from build123d import *

# Parameters (mm, degrees)
F1_DEPTH = 1600
F2_R     = 4.5
F3_DEPTH = 40.001


with BuildPart() as f1:
    # F0 (on Top) → F1 (new body)
    with BuildSketch(Plane.XY):
        with BuildLine():
            Line((-15.5, -20), (15.5, -20))
            ThreePointArc((15.5, -20), (18.681981, -18.681981), (20, -15.5))
            Line((20, -15.5), (20, 15.5))
            ThreePointArc((20, 15.5), (18.681981, 18.681981), (15.5, 20))
            Line((15.5, 20), (-15.5, 20))
            ThreePointArc((-15.5, 20), (-18.681981, 18.681981), (-20, 15.5))
            Line((-20, 15.5), (-20, -15.5))
            ThreePointArc((-20, -15.5), (-18.681981, -18.681981), (-15.5, -20))
        make_face()
        with BuildLine():
            ThreePointArc((15.5, 17), (16.56066, 16.56066), (17, 15.5))
            Line((17, 15.5), (17, -15.5))
            ThreePointArc((17, -15.5), (16.56066, -16.56066), (15.5, -17))
            Line((15.5, -17), (-15.5, -17))
            ThreePointArc((-15.5, -17), (-16.56066, -16.56066), (-17, -15.5))
            Line((-17, -15.5), (-17, 15.5))
            ThreePointArc((-17, 15.5), (-16.56066, 16.56066), (-15.5, 17))
            Line((-15.5, 17), (15.5, 17))
        make_face(mode=Mode.SUBTRACT)
    extrude(amount=F1_DEPTH)

    # F2 (on face) → F3 (cut, through all)
    with BuildSketch(Plane.YZ.offset(20)):
        with Locations((0, 1540)):
            Circle(F2_R)
        with Locations((0, 60)):
            Circle(F2_R)
    extrude(amount=-F3_DEPTH, mode=Mode.SUBTRACT)


solid = f1.part
Check sheet for the modelled part. Datum: model origin and axes. Units: mm. A direction names the side the tool comes from. Give positions to 0.01 mm unless a question says otherwise; leave off trailing zeros. Loops run counter-clockwise (first coordinate to the right, second up) from the corner with the lowest first, then second, coordinate; pieces in that order, holes last. Notation, with made-up numbers: M 38,57 L 81,57 A21 cw 81,91 Z; hole C 84,-34 d7. An arc over 180 degrees is marked long. Answer as a JSON object with one key per item and string values. Group by question number.
Q1. Cross-section at A-A on x = 8.5. Record the cut outline in (y, z), then the cut area to 3 significant figures.
Q2. Material ranges on line 1 along Z through (x, y) = (17.9, 0); line 2 along X through (y, z) = (-5, 1138.5), recorded low to high. Write a range as [from, to].
Q3. Access from +Z, -Z, +X, -X, +Y, -Y to the whole of each face (thin tool, end or side, straight path). Record for faces 1 (the flat face through (17, 0, 789)), 2 (the flat face through (-20, 0, 789)).
Q4. Release check for a two-part mould opening along X. For faces 3 (the flat face through (0, -17, 789)), 4 (the flat face through (0, 20, 789)), 5 (the flat face through (20, 0, 789)) record: released by +X, released by -X, zero draft, split by the parting line, or undercut.
Q5. Cross-section at B-B on z = 862.5. Record the cut outline in (x, y), then the cut area to 3 significant figures.
Evaluation:
{
 "1": {"outline": "M -20,0 L -17,0 L -17,1600 L -20,1600 Z; M 17,0 L 20,0 L 20,1600 L 17,1600 Z", "area": "9,600 mm2"},
 "2": {"line 1": "z = [0, 55.5], [64.5, 1535.5], [1544.5, 1600]", "line 2": "x = [-20, -17], [17, 20]"},
 "3": {"face 1": "+Z, -Z", "face 2": "+Z, -Z, -X, +Y, -Y"},
 "4": {"face 3": "undercut", "face 4": "zero draft", "face 5": "released by +X"},
 "5": {"outline": "M -20,-15.5 A4.5 ccw -15.5,-20 L 15.5,-20 A4.5 ccw 20,-15.5 L 20,15.5 A4.5 ccw 15.5,20 L -15.5,20 A4.5 ccw -20,15.5 Z; hole M -17,-15.5 A1.5 ccw -15.5,-17 L 15.5,-17 A1.5 ccw 17,-15.5 L 17,15.5 A1.5 ccw 15.5,17 L -15.5,17 A1.5 ccw -17,15.5 Z", "area": "429 mm2"}
}
